For this review, take the finished solid that the model builds, in its own axes (mm). Face numbers are marked on the shaded views. Coordinates: 2 decimals unless noted, no trailing zeros. Order: outer loops, then holes, each group sorted by start corner. A loop starts at its lowest first (then second) coordinate and runs counter-clockwise, first axis right, second up.
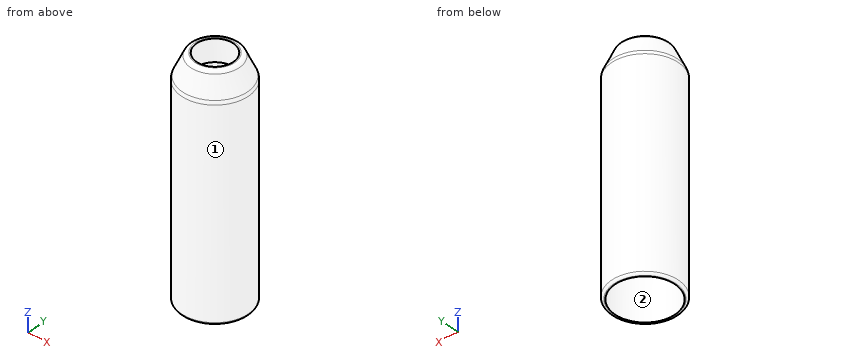
from build123d import *

# Parameters (mm, degrees)
F3_R = 2
F4_R = 4
F5_R = 1


with BuildPart() as f2:
    # F0 (on Front) → F2 (revolve)
    with BuildSketch(Plane.XZ):
        Polygon((10, 95.136816), (8, 95.02412), (8.562585, 85.039958), (13.062585, 85.039958), (13.062585, -4.960042), (14.562585, -4.960042), (14.562585, 85.039958), align=None)
    revolve(axis=Axis((0, 0, 47.995005), (0, 0, 1)))

    # F3
    f3_edges = [f2.edges().sort_by_distance(p)[0] for p in [
        (-10, 0, 95.136816),
    ]]
    fillet(f3_edges, radius=F3_R)

    # F4
    f4_edges = [f2.edges().sort_by_distance(p)[0] for p in [
        (-14.562585, 0, 85.039958),
    ]]
    fillet(f4_edges, radius=F4_R)

    # F5
    f5_edges = [f2.edges().sort_by_distance(p)[0] for p in [
        (-14.562585, 0, -4.960042),
    ]]
    fillet(f5_edges, radius=F5_R)


solid = f2.part
1. Take a section at A-A, the plane z = 63.5. Give the boundary of the cut face in (x, y).
Answer below:
outline: circle Ø29.13 at (0, 0); hole circle Ø26.13 at (0, 0)
2. Take a section at B-B, the plane z = 87. Give the boundary of the cut face in (x, y).
Answer below:
outline: circle Ø27.35 at (0, 0); hole circle Ø16.9 at (0, 0)
3. The part is to be moulded in two halves that separate along Y. For the marked faces 1 and 2, say which applies: +Y half, -Y half, draft (parallel to the pull), parting line (faces both ways), or undercut.
Answer below:
face 1: parting line
face 2: undercut
4. Clearance check with flat-ended pins moving along their axes: pin 1 Ø5 at (y, z) = (10, 63) entering from -X; pin 2 Ø4 at (x, y) = (7, -8) entering from -Z; pin 3 Ø1 at (y, z) = (2, 80.5) entering from -X. State where each tip first meets the part, or that it passes through.
Answer below:
pin 1: stops at x = -12.48
pin 2: stops at z = 85.04
pin 3: stops at x = -14.49
5. To check wall thickness, follow L1, parallel to Y at x = 0, z = 26; L2, parallel to X at y = 4.5, z = 62.5; L3, parallel to Y at x = -6.5, z = 47.5. State the ranges of each line that lie inside material, in increasing order.
Answer below:
L1: y = -14.56 to -13.06, 13.06 to 14.56
L2: x = -13.85 to -12.26, 12.26 to 13.85
L3: y = -13.03 to -11.33, 11.33 to 13.03
